Part model, mm, in its own coordinate system. A direction names the side the tool comes from. Round coordinates to 2 decimals unless told otherwise and drop trailing zeros. Loops run counter-clockwise (first coordinate to the right, second up) from the corner with the lowest first, then second, coordinate; pieces in that order, holes last. Notation, with made-up numbers: M 83.5,26 L 96.5,26 A24 ccw 96.5,56 Z; hole C 64,36.25 d5. An arc over 180 degrees is marked long. Put each result on its own line as item: value. Start each with the question number.
1) Slice it at B-B on x = 0. Give the cut face in (y, z) (3 decimals), then the cut area to 3 significant figures.
2) Drop flat-ended pins along their axis: pin 1 Ø3 at (x, y) = (6.5, 14) entering from -Z; pin 2 Ø3 at (x, y) = (3, 17) entering from -Z; pin 3 Ø7 at (y, z) = (16.5, -3) entering from +X. Give the stop position or say it passes through.
3) Slice it at A-A on z = -4. Give the cut face in (x, y).
4) Pull direction X, two halves, no side cores. Call faces 1 (the cylindrical face through (-7.95, 0.09, -36.87)), 2 (the flat face through (0, 17, 0.7)), 3 (the flat face through (-16.5, 0, -14)): +X half, -X half, draft (parallel to the pull), parting line (faces both ways), or undercut.
5) Slice it at C-C on z = 10.5. Give the cut face in (x, y).
6) Which spindle directions (+Z, -Z, +X, -X, +Y, -Y) get a long thin tool onto all of the face, cutting with end or side? Do faces 4 (the flat face through (0, 14.3, 11)), 5 (the flat face through (-11, 5.35, -14)), 6 (the flat face through (-7.5, 20, -2)), 7 (the flat face through (15, 0, 0)), 8 (the flat face through (-13.5, 0, 12)). Say none if no direction does.
7) Probe line 1 along X through (y, z) = (20, -10); line 2 along Z through (x, y) = (-11.5, -2.5); line 3 along Y through (x, z) = (-2.5, 22). List the from-to ranges inside material, lowest first.
8) Slice it at D-D on y = 10. Give the cut face in (x, z).
```python
from build123d import *

# Parameters (mm, degrees)
SKETCH1_W           = 27
SKETCH1_H           = 28
BOSS_EXTRUDE1_DEPTH = 25
SKETCH2_W           = 33
SKETCH2_H           = 10.7
SKETCH2_W_2         = 10.5
SKETCH2_H_2         = 28
BOSS_EXTRUDE2_DEPTH = 28
SKETCH3_R           = 2.05
BOSS_EXTRUDE3_DEPTH = 18
EXTRUDE_THIN1_DEPTH = 7.5
MOUNTING_HOLE_REACH = 61.705
SKETCH5_R           = 3.075


with BuildPart() as part:
    # Sketch1 → Boss-Extrude1 (new body)
    with BuildSketch(Plane.XY):
        Rectangle(SKETCH1_W, SKETCH1_H)
    extrude(amount=BOSS_EXTRUDE1_DEPTH)

    # Sketch2 → Boss-Extrude2 (add)
    with BuildSketch(Plane.XY):
        Rectangle(SKETCH2_W, SKETCH2_H)
        Rectangle(SKETCH2_W_2, SKETCH2_H_2)
    extrude(amount=-BOSS_EXTRUDE2_DEPTH)

    # Sketch3 → Boss-Extrude3 (add)
    with BuildSketch(Plane(origin=(0, 0, -28), x_dir=(-1, 0, 0), z_dir=(0, 0, -1))):
        with Locations((-10, 0)):
            Circle(SKETCH3_R)
        with Locations((10, 0)):
            Circle(SKETCH3_R)
        with Locations((0, 10)):
            Circle(SKETCH3_R)
        with Locations((0, -10)):
            Circle(SKETCH3_R)
    extrude(amount=BOSS_EXTRUDE3_DEPTH)

    # Sketch4 → Extrude-Thin1 (add, symmetric)
    with BuildSketch(Plane(origin=(0, 0, 0), x_dir=(0, 0, -1), z_dir=(1, 0, 0))):
        with BuildLine():
            Line((-19.356513239, 13.7), (-2.349136171, 13.7))
            ThreePointArc((-2.349136171, 13.7), (-1.303107706, 14.059916252), (-0.7, 14.987265351))
            Line((-0.7, 14.987265351), (-0.7, 18.658359214))
            ThreePointArc((-0.7, 18.658359214), (-0.494115365, 19.29910699), (0.04646857, 19.7))
            Line((0.04646857, 19.7), (16, 19.7))
            Line((16, 19.7), (16, 20.3))
            Line((16, 20.3), (-0.041605625, 20.3))
            ThreePointArc((-0.041605625, 20.3), (-0.949208947, 19.692590918), (-1.3, 18.658359214))
            Line((-1.3, 18.658359214), (-1.3, 15.069374388))
            ThreePointArc((-1.3, 15.069374388), (-1.698631818, 14.512957675), (-2.349136171, 14.3))
            Line((-2.349136171, 14.3), (-19.356513239, 14.3))
            Line((-19.356513239, 14.3), (-19.356513239, 13.7))
        make_face()
    extrude(amount=EXTRUDE_THIN1_DEPTH, both=True)

    # Sketch5 → Mounting Hole (cut, up to next)
    with BuildSketch(Plane(origin=(0, 20.3, 0), x_dir=(1, 0, 0), z_dir=(0, 1, 0)), mode=Mode.PRIVATE) as mounting_hole_sk1:
        with Locations(Location((0, 10.2, 0), (0, 0, 270))):
            Circle(SKETCH5_R)
    mounting_hole_tool1 = extrude(mounting_hole_sk1.sketch, amount=-MOUNTING_HOLE_REACH, mode=Mode.PRIVATE) & part.part
    add(mounting_hole_tool1.solids().sort_by_distance((0, 20.3, -10.2))[0], mode=Mode.SUBTRACT)


solid = part.part
```
Recorded:
1. outline: M -14,-28 L -12.05,-28 L -12.05,-46 L -7.95,-46 L -7.95,-28 L 7.95,-28 L 7.95,-46 L 12.05,-46 L 12.05,-28 L 14,-28 L 14,1.385 A1.7 ccw 14.987,0.7 L 18.658,0.7 A1.1 cw 19.7,-0.046 L 19.7,-7.125 L 20.3,-7.125 L 20.3,0.042 A1.7 ccw 18.658,1.3 L 15.069,1.3 A1.1 cw 14.3,2.349 L 14.3,19.357 L 14,19.357 L 14,25 L -14,25 Z; M 19.7,-16 L 20.3,-16 L 20.3,-13.275 L 19.7,-13.275 Z
1. area: 1,650 mm2
2. pin 1: stops at z = -28
2. pin 2: stops at z = 0.7
2. pin 3: stops at x = 7.5
3. outline: M -16.5,-5.35 L -5.25,-5.35 L -5.25,-14 L 5.25,-14 L 5.25,-5.35 L 16.5,-5.35 L 16.5,5.35 L 5.25,5.35 L 5.25,14 L -5.25,14 L -5.25,5.35 L -16.5,5.35 Z; M -7.5,19.7 L 7.5,19.7 L 7.5,20.3 L -7.5,20.3 Z
4. face 1: undercut
4. face 2: draft
4. face 3: -X half
5. outline: M -13.5,-14 L 13.5,-14 L 13.5,14 L 7.5,14 L 7.5,14.3 L -7.5,14.3 L -7.5,14 L -13.5,14 Z
6. face 4: +Z, +X, -X, +Y
6. face 5: -Z, -X
6. face 6: +Z, -Z, -X, +Y
6. face 7: +Z, +X, +Y, -Y
6. face 8: +Z, -X, +Y, -Y
7. line 1: x = -7.5 to -3.07, 3.07 to 7.5
7. line 2: z = -28 to 25
7. line 3: y = -14 to 14
8. outline: M -13.5,0 L -5.25,0 L -5.25,-28 L -2.05,-28 L -2.05,-46 L 2.05,-46 L 2.05,-28 L 5.25,-28 L 5.25,0 L 13.5,0 L 13.5,25 L -13.5,25 Z
